Build history of the part. All positions in model axes, mm. Round coordinates to 2 decimals unless told otherwise and drop trailing zeros. Loops run counter-clockwise (first coordinate to the right, second up) from the corner with the lowest first, then second, coordinate; pieces in that order, holes last. Notation, with made-up numbers: (49, -6.75) - (70, -6.75) arc R7 ccw to (70, 2.25) - close; hole circle Ø11 at (47, 84). An arc over 180 degrees is marked (long way). Use one line per item in the form item = value. Start each with the question number.
Q1. Mould opens along Y. For faces 1 (the face through (66, 130, 5)), 2 (the face through (14.77, 121.5, 5.07)), 3 (the face through (0, 66, 5)) say: released by +Y, released by -Y, zero draft, split by the parting line, or undercut.
Q2. Saw through at C-C (z = 6.75). Count the separate pieces of the cut face and the enclosed holes in it, then the cut area to 3 significant figures.
Q3. Saw through at A-A (y = 10). Give the cut face in (x, z), then the cut area to 3 significant figures.
Q4. Pin check, flat tips, straight feed: pin 1 (16 mm diameter, centred on x = 10, y = 10, fed in from +Z); pin 2 (6 mm diameter, centred on x = 10, y = 120, fed in from -Z). Stop position of each tip, or through.
Q5. Drill centre lines: line 1 (Y direction, x = 120, z = 5.5); line 2 (Y direction, x = 121, z = 5). Where is each one in solid material? Low to high.
Autodesk Inventor part; units mm, degrees
ref_plane "YZ Plane" through (0, 0, 0) normal (1, 0, 0) x (0, 1, 0)
ref_plane "XZ Plane" through (0, 0, 0) normal (0, 1, 0) x (-1, 0, 0)
ref_plane "XY Plane" through (0, 0, 0) normal (0, 0, 1) x (1, 0, 0)
sketch "Sketch1" plane through (0, 0, 0) normal (0, 0, 1) x (1, 0, 0)
  line L0 (0, 0) -> (130, 0)
  line L1 (130, 0) -> (130, 130)
  line L2 (130, 130) -> (0, 130)
  line L3 (0, 130) -> (0, 0)
  dimension "d0" = 130
  dimension "d1" = 130
extrude "Extrusion1" add sketch "Sketch1" along normal blind 10
sketch "Sketch2" plane through (0, 0, 10) normal (0, 0, 1) x (1, 0, 0)
  line L0 (0, 0) -> (130, 0)
  line L1 (0, 0) -> (10, 0)
  line L2 (10, 0) -> (10, 110)
  line L3 (10, 110) -> (10, 120)
  line L4 (10, 120) -> (120, 120)
  line L5 (120, 120) -> (120, 10)
  line L6 (120, 10) -> (10, 10)
  circle A0 centre (10, 120) radius 5
  circle A1 centre (120, 120) radius 5
  circle A2 centre (10, 10) radius 5
  circle A3 centre (120, 10) radius 5
  dimension "d4" = 10
  dimension "d5" = 110
  dimension "d6" = 10
  dimension "d7" = 110
  dimension "d8" = 110
  dimension "d9" = 110
  dimension "d10" = 10
  dimension "d11" = 10
  dimension "d12" = 10
  dimension "d13" = 10
extrude "Extrusion2" cut sketch "Sketch2" against normal through all contours A2 L2 | L2 L6 A2 | L2 A2 L6 | A3 L5 L6 | L6 L5 A3 | A0 L4 L3 | L3 L4 A0 | A1 L4 L5 | L5 L4 A1
sketch "Sketch3" plane through (0, 0, 10) normal (0, 0, 1) x (1, 0, 0)
  line L0 (0, 0) -> (130, 0)
  line L1 (68.2625, 0) -> (63.2625, 0)
  line L2 (63.2625, 0) -> (63.2625, 5)
  circle A0 centre (63.2625, 5) radius 0.05
  dimension "d16" = 5
  dimension "d17" = 5
  dimension "d18" = 0.1
extrude "Extrusion3" cut sketch "Sketch3" along normal through all both and the other way through all
sketch "Sketch4" plane through (0, 0, 10) normal (0, 0, 1) x (1, 0, 0)
  line L0 (63.5, 131.7625) -> (63.5, 126.7625)
  circle A0 centre (63.5, 126.7625) radius 0.05
  point P0 (0, 0)
  dimension "d21" = 5
  dimension "d22" = 0.1
extrude "Extrusion4" cut sketch "Sketch4" against normal blind 10
sketch "Sketch5" plane through (0, 0, 10) normal (0, 0, 1) x (1, 0, 0)
  line L0 (0, 63.5) -> (5, 63.5)
  line L1 (5, 63.5) -> (123.825, 63.5)
  circle A0 centre (5, 63.5) radius 0.5
  circle A1 centre (123.825, 63.5) radius 0.5
  point P0 (0, 0)
  dimension "d25" = 5
  dimension "d26" = 1
  dimension "d27" = 1
extrude "Extrusion5" cut sketch "Sketch5" against normal through all
sketch "Sketch6" plane through (0, 0, 10) normal (0, 0, 1) x (1, 0, 0)
  point P0 (0, 0)
properties part number "STAND PLATE FOR STORSGE SYSTEM"
Report:
q1.face_1 = released by +Y
q1.face_2 = undercut
q1.face_3 = zero draft
q2.separate_pieces = 1
q2.enclosed_holes = 8
q2.area = 16,600 mm²
q3.outline = (0, 0) - (5, 0) - (5, 10) - (0, 10) - close; (15, 0) - (115, 0) - (115, 10) - (15, 10) - close; (125, 0) - (130, 0) - (130, 10) - (125, 10) - close
q3.area = 1,100 mm²
q4.pin_1 = 10
q4.pin_2 = through
q5.line_1 = 0 to 5, 15 to 115, 125 to 130
q5.line_2 = 0 to 5.1, 14.9 to 115.1, 124.9 to 130
